CAD build for the part. Positions are in the model's coordinates, mm. Face numbers are marked on the shaded views. A direction names the side the tool comes from. Coordinates: 2 decimals unless noted, no trailing zeros. Order: outer loops, then holes, each group sorted by start corner. A loop starts at its lowest first (then second) coordinate and runs counter-clockwise, first axis right, second up. Notation, with made-up numbers: M 44.25,29.25 L 89.25,29.25 A32 ccw 89.25,67.25 Z; hole C -9.75,42 d11. An arc over 180 degrees is marked long. One line per item, written item: value.
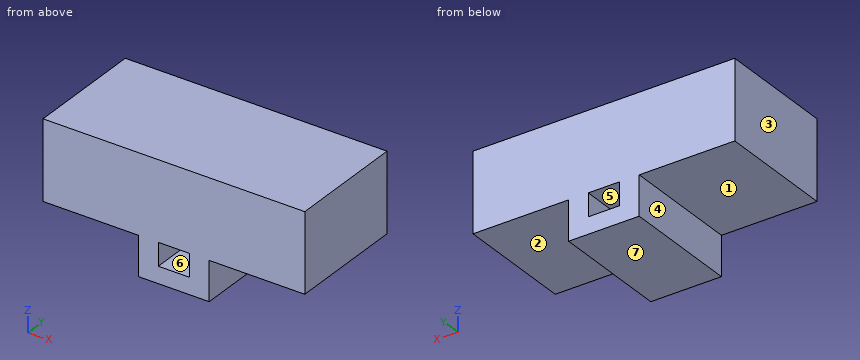
from build123d import *

# Parameters (mm, degrees)
SKETCH008_W      = 1.5
SKETCH008_H      = 1.1
EXTRUDE008_DEPTH = 5.7
BOX004_W         = 4.6
BOX004_H         = 5.7
BOX004_DEPTH     = 1.9
BOX003_W         = 4.6
BOX003_H         = 5.7
BOX003_DEPTH     = 1.9
BOX002_W         = 12.6
BOX002_H         = 5.7
BOX002_DEPTH     = 5.7


with BuildPart() as extrude008:
    # Sketch008 (on Sketch) → Extrude008 (new body)
    with BuildSketch(Plane.XZ):
        with Locations((6.3, 2.15)):
            Rectangle(SKETCH008_W, SKETCH008_H)
    extrude(amount=-EXTRUDE008_DEPTH)


with BuildPart() as cube004:
    # Box004 → Box004 (new body)
    with BuildSketch(Plane(origin=(8, 0, 0.8), x_dir=(1, 0, 0), z_dir=(0, 0, 1))):
        with Locations((2.3, 2.85)):
            Rectangle(BOX004_W, BOX004_H)
    extrude(amount=BOX004_DEPTH)


with BuildPart() as cube003:
    # Box003 → Box003 (new body)
    with BuildSketch(Plane.XY.offset(0.8)):
        with Locations((2.3, 2.85)):
            Rectangle(BOX003_W, BOX003_H)
    extrude(amount=BOX003_DEPTH)


with BuildPart() as cut015:
    # Box002 → Box002 (new body)
    with BuildSketch(Plane.XY.offset(0.8)):
        with Locations((6.3, 2.85)):
            Rectangle(BOX002_W, BOX002_H)
    extrude(amount=BOX002_DEPTH)

    # Cut: cut Cube003
    add(cube003.part, mode=Mode.SUBTRACT)

    # Cut001: cut Cube004
    add(cube004.part, mode=Mode.SUBTRACT)

    # Cut015: cut Extrude008
    add(extrude008.part, mode=Mode.SUBTRACT)


solid = cut015.part
Q1. Mould opens along Z. For the marked faces 4, 5, 6 and 7 say: released by +Z, released by -Z, zero draft, split by the parting line, or undercut.
Recorded:
face 4: zero draft
face 5: undercut
face 6: undercut
face 7: released by -Z
Q2. Pin check, flat tips, straight feed: pin 1 Ø2 at (y, z) = (3.5, 2) entering from -X; pin 2 Ø1.5 at (y, z) = (1.5, 1.5) entering from +X; pin 3 Ø0.9 at (y, z) = (3.5, 2) entering from -X; pin 4 Ø2 at (x, y) = (10.5, 5) entering from -Z. Stop position of each tip, or through.
Recorded:
pin 1: stops at x = 0
pin 2: stops at x = 8
pin 3: stops at x = 4.6
pin 4: stops at z = 2.7
Q3. Drill centre lines: line 1 along X through (y, z) = (2.6, 2.6); line 2 along Z through (x, y) = (10.5, 2.8); line 3 along X through (y, z) = (3.55, 1.5). Where is each one in solid material? Low to high.
Recorded:
line 1: x = 4.6 to 5.55, 7.05 to 8
line 2: z = 2.7 to 6.5
line 3: x = 4.6 to 8
Q4. Slice it at C-C (y = 3.2). List the corners of the cut face in (x, z), plus the area to 3 significant figures.
Recorded:
outline: M 0,2.7 L 4.6,2.7 L 4.6,0.8 L 8,0.8 L 8,2.7 L 12.6,2.7 L 12.6,6.5 L 0,6.5 Z; hole M 5.55,1.6 L 7.05,1.6 L 7.05,2.7 L 5.55,2.7 Z
area: 52.7 mm^2
Q5. Which spindle directions (+Z, -Z, +X, -X, +Y, -Y) get a long thin tool onto all of the face, cutting with end or side? Do the marked faces 1, 2 and 3. Say none if no direction does.
Recorded:
face 1: -Z, -X, +Y, -Y
face 2: -Z, +X, +Y, -Y
face 3: +Z, -Z, -X, +Y, -Y
Q6. Slice it at A-A (z = 1.95). List the corners of the cut face in (x, y), plus the area to 3 significant figures.
Recorded:
outline: M 4.6,0 L 5.55,0 L 5.55,5.7 L 4.6,5.7 Z; M 7.05,0 L 8,0 L 8,5.7 L 7.05,5.7 Z
area: 10.8 mm^2
Q7. Slice it at D-D (x = 9.75). List the corners of the cut face in (y, z), plus the area to 3 significant figures.
Recorded:
outline: M 0,2.7 L 5.7,2.7 L 5.7,6.5 L 0,6.5 Z
area: 21.7 mm^2
Q8. Slice it at B-B (x = 6.75). List the corners of the cut face in (y, z), plus the area to 3 significant figures.
Recorded:
outline: M 0,0.8 L 5.7,0.8 L 5.7,1.6 L 0,1.6 Z; M 0,2.7 L 5.7,2.7 L 5.7,6.5 L 0,6.5 Z
area: 26.2 mm^2
